Design review of the part shown in the three views and the two pictorial views. Dimensions are in mm from the part's minimum x, y and z. A direction names the side the tool comes from. Round coordinates to 2 decimals unless told otherwise and drop trailing zeros. Order: outer loops, then holes, each group sorted by start corner. A loop starts at its lowest first (then second) coordinate and runs counter-clockwise, first axis right, second up. Notation, with made-up numbers: (-34.75, 2) - (-9.75, 2) arc R15 cw to (-9.75, 13) - close; hole circle Ø5 at (68, -28). An arc over 180 degrees is marked (long way). Use CSV: the item, a comma, the result in double quotes.
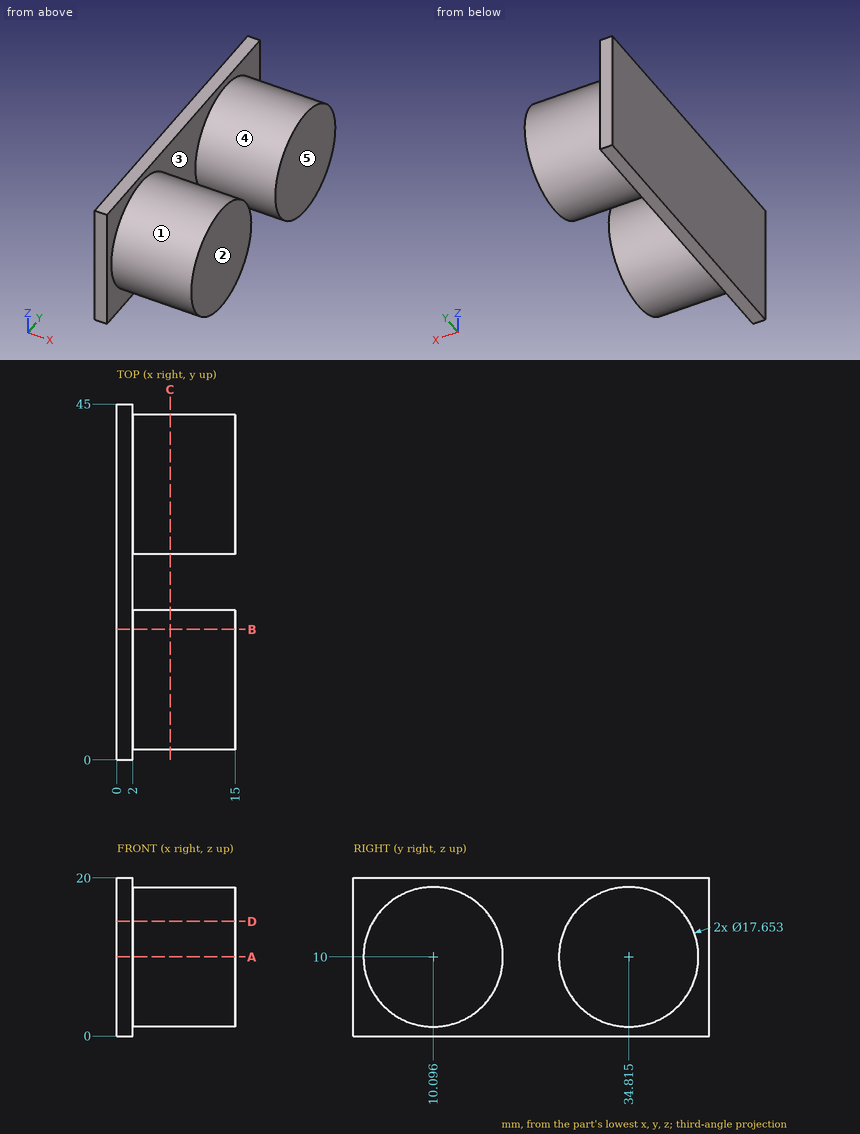
1) To check wall thickness, follow L1, parallel to Y at x = 10, z = 16.5 (1 decimal); L2, parallel to Y at x = 8, z = 13.25; L3, parallel to X at y = 25.5, z = 4. State the ranges of each line that lie inside material, in increasing order. Write a range as from..to.
Data:
L1,"y = 4.1..16.1, 28.8..40.8"
L2,"y = 1.89..18.3, 26.61..43.02"
L3,"x = 0..2"
2) Insertion check: pin 1 Ø4 at (x, z) = (5, 15) entering from +Y (1 decimal); pin 2 Ø1 at (x, y) = (7.5, 7) entering from -Z (1 decimal); pin 3 Ø2 at (x, y) = (5, 7.5) entering from +Z. Each pin has a flat end and moves straight along its axis. Give the tip position at first contact, or say it passes through.
Data:
pin 1,"stops at y = 43.1"
pin 2,"stops at z = 1.6"
pin 3,"stops at z = 18.68"
3) We need section C-C (x = 6.75). Give the boundary of the cut face in (y, z) (1 decimal).
Data:
outline,"circle Ø17.7 at (10.1, 10); circle Ø17.7 at (34.8, 10)"
4) The part is to be moulded in two halves that separate along Y. For the marked faces 1, 2 and 3, say which applies: +Y half, -Y half, draft (parallel to the pull), parting line (faces both ways), or undercut.
Data:
face 1,"undercut"
face 2,"draft"
face 3,"undercut"
5) For the marked faces 4 and 5, list the 3-axis set-ups (+Z, -Z, +X, -X, +Y, -Y) from which the entire face can be reached by the end or side of a thin tool; tool diameter is ignored.
Data:
face 4,"+X"
face 5,"+Z, -Z, +X, +Y, -Y"
6) We need section D-D (z = 14.5). Give the boundary of the cut face in (x, y).
Data:
outline,"(0, 0) - (2, 0) - (2, 2.5) - (15, 2.5) - (15, 17.69) - (2, 17.69) - (2, 27.22) - (15, 27.22) - (15, 42.41) - (2, 42.41) - (2, 45) - (0, 45) - close"
7) We need section A-A (z = 10). Give the boundary of the cut face in (x, y).
Data:
outline,"(0, 0) - (2, 0) - (2, 1.27) - (15, 1.27) - (15, 18.92) - (2, 18.92) - (2, 25.99) - (15, 25.99) - (15, 43.64) - (2, 43.64) - (2, 45) - (0, 45) - close"
8) We need section B-B (y = 16.5). Give the boundary of the cut face in (x, z) (1 decimal), then the cut area to 3 significant figures.
Data:
outline,"(0, 0) - (2, 0) - (2, 3.9) - (15, 3.9) - (15, 16.1) - (2, 16.1) - (2, 20) - (0, 20) - close"
area,"198 mm2"
